Geometry check sheet. Reference: drawing and pictorial views, mm from the part's lowest x, y, z. Give positions to 0.01 mm unless a question says otherwise; leave off trailing zeros. Loops run counter-clockwise (first coordinate to the right, second up) from the corner with the lowest first, then second, coordinate; pieces in that order, holes last. Notation, with made-up numbers: (16.5, 58.25) -> (68.5, 58.25) arc R22 cw to (68.5, 81.25) -> close; hole circle Ø6 at (-21, -0.75). An arc over 180 degrees is marked (long way). One line per item, written item: value. Start each with the question number.
(1) Scan lines: line 1 along Z through (x, y) = (11.5, 0.5) (1 decimal); line 2 along X through (y, z) = (0.35, 125.5) (1 decimal); line 3 along Z through (x, y) = (15.5, 3.2) (1 decimal). Record each from-to range of solid material in increasing order. Write a range as from..to.
(2) Sectioned sample at C-C, the plane y = 2.9. State how many separate pieces and enclosed holes the cut face has, then the cut area to 3 significant figures.
(3) Gauge pin test, flat ends, axial feed: pin 1 Ø2 at (y, z) = (1.5, 32) entering from -X; pin 2 Ø1.5 at (y, z) = (2.5, 110.5) entering from +X. Record the tip position at first contact, or that the pin passes through.
(4) Sectioned sample at D-D, the plane z = 37. Record the cut outline in (x, y), then the cut area to 3 significant figures.
(5) Sectioned sample at B-B, the plane z = 10. Record the cut outline in (x, y), then the cut area to 3 significant figures.
(6) Sectioned sample at A-A, the plane x = 40. Record the cut outline in (y, z) (1 decimal), then the cut area to 3 significant figures.
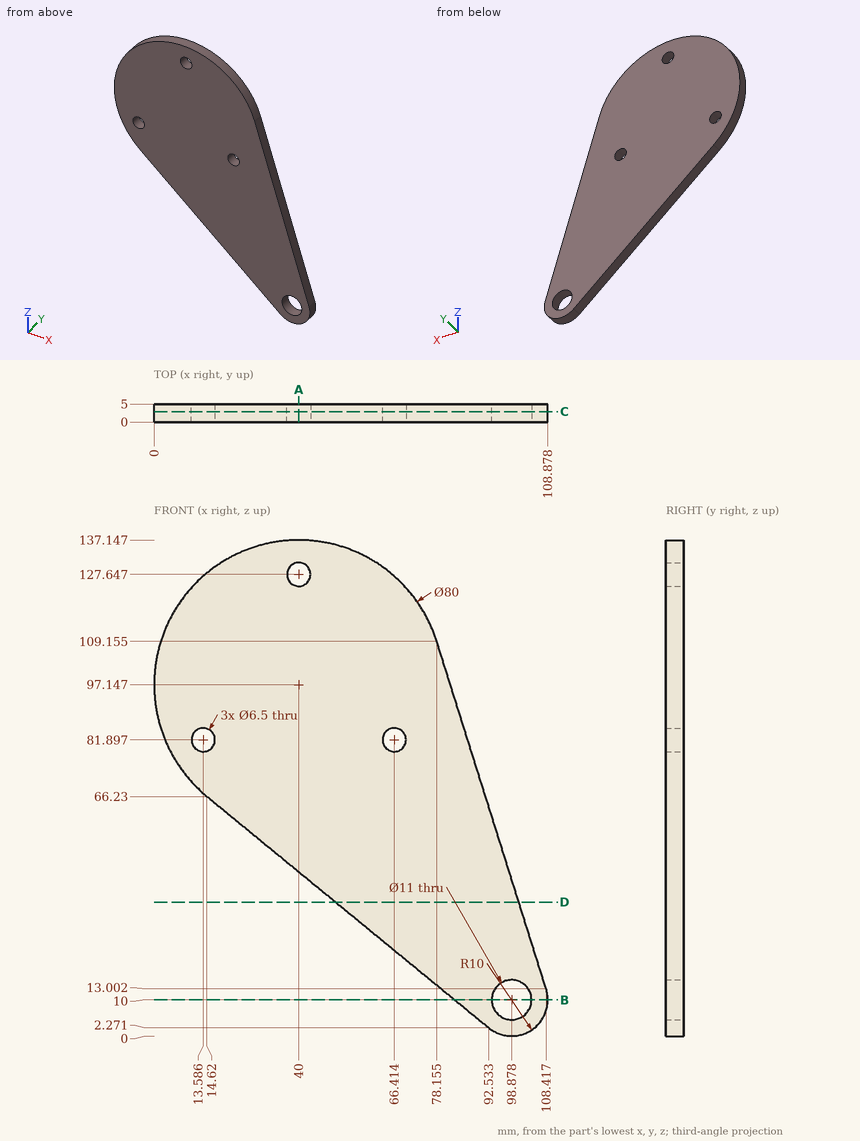
Calculated:
1. line 1: z = 69.1..79.4, 84.4..125.2
1. line 2: x = 11.8..37.6, 42.4..68.2
1. line 3: z = 65.5..79.3, 84.5..128.8
2. separate pieces: 1
2. enclosed holes: 4
2. area: 7,950 mm2
3. pin 1: stops at x = 55.1
3. pin 2: stops at x = 77.96
4. outline: (50.23, 0) -> (100.86, 0) -> (100.86, 5) -> (50.23, 5) -> close
4. area: 253 mm2
5. outline: (83.12, 0) -> (93.38, 0) -> (93.38, 5) -> (83.12, 5) -> close; (104.38, 0) -> (108.88, 0) -> (108.88, 5) -> (104.38, 5) -> close
5. area: 73.8 mm2
6. outline: (0, 45.4) -> (5, 45.4) -> (5, 124.4) -> (0, 124.4) -> close; (0, 130.9) -> (5, 130.9) -> (5, 137.1) -> (0, 137.1) -> close
6. area: 426 mm2
